```python
from build123d import *

# Parameters (mm, degrees)
F0_R     = 11.75
F1_DEPTH = 1.5
F2_R     = 0.5
F3_R     = 4
F4_DEPTH = 3.5
F5_R     = 5.75
F6_DEPTH = 0.5


with BuildPart() as f1:
    # F0 (on Top) → F1 (new body)
    with BuildSketch(Plane.XY):
        Circle(F0_R)
    extrude(amount=-F1_DEPTH)

    # F2
    f2_edges = [f1.edges().sort_by_distance(p)[0] for p in [
        (-11.75, 0, 0),
    ]]
    fillet(f2_edges, radius=F2_R)

    # F3 (on face) → F4 (join)
    with BuildSketch(Plane(origin=(0, 0, -1.5), x_dir=(1, 0, 0), z_dir=(0, 0, -1))):
        Circle(F3_R)
    extrude(amount=F4_DEPTH)

    # F5 (on face) → F6 (join)
    with BuildSketch(Plane(origin=(0, 0, -1.5), x_dir=(1, 0, 0), z_dir=(0, 0, -1))):
        Circle(F5_R)
    extrude(amount=F6_DEPTH)


solid = f1.part
```
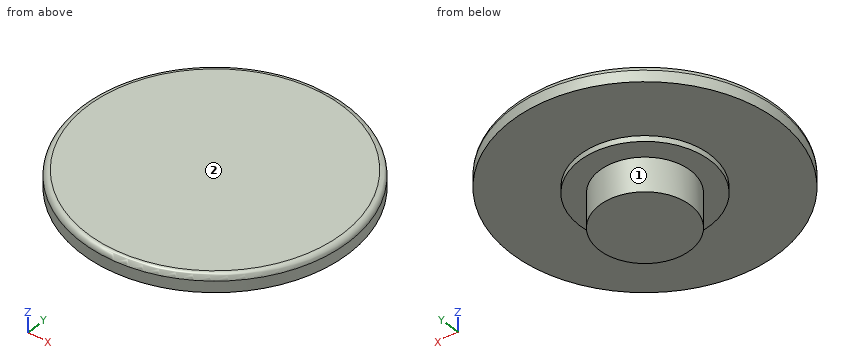
Read the model definition and answer for the solid it produces. Units are mm, in the model's axes. Face numbers are marked on the shaded views. A direction names the side the tool comes from. Round coordinates to 2 decimals unless told otherwise and drop trailing zeros. Write each loop counter-clockwise with the first axis right and the second up, starting at its lowest first coordinate (ties: lowest second). Pieces come first, ordered by that corner, then holes. Notation, with made-up numbers: (-25.5, 57.5) - (-3.5, 57.5) arc R35 cw to (-3.5, 95.5) - close; hole circle Ø3 at (32, 33). An arc over 180 degrees is marked (long way). One line per item, written item: value.
Q1. This flat-tipped pin is pushed along its axis until it touches: P1, Ø1, axis at x = -2, z = -4, coming from the -Y side. Where does it stop, or does it pass through?
The answers:
P1: stops at y = -3.71
Q2. Find section A-A (x = 0). Determine the outline of the cut face in (y, z).
The answers:
outline: (-11.75, -1.5) - (-5.75, -1.5) - (-5.75, -2) - (-4, -2) - (-4, -5) - (4, -5) - (4, -2) - (5.75, -2) - (5.75, -1.5) - (11.75, -1.5) - (11.75, -0.5) arc R0.5 ccw to (11.25, 0) - (-11.25, 0) arc R0.5 ccw to (-11.75, -0.5) - close
Q3. Straight lines are drawn through the part: line 1 (Z direction, x = -1, y = 10); line 2 (X direction, y = 0.25, z = -0.9); line 3 (Y direction, x = -8, z = -1.4). For each, find the intervals that lie inside material, in ascending order. Write a range as from..to.
The answers:
line 1: z = -1.5..0
line 2: x = -11.75..11.75
line 3: y = -8.61..8.61
Q4. Which of the six approach directions +Z, -Z, +X, -X, +Y, -Y give full straight-line access (tool end or side, diameter ignored) to the marked faces 1 and 2?
The answers:
face 1: -Z
face 2: +Z, +X, -X, +Y, -Y
